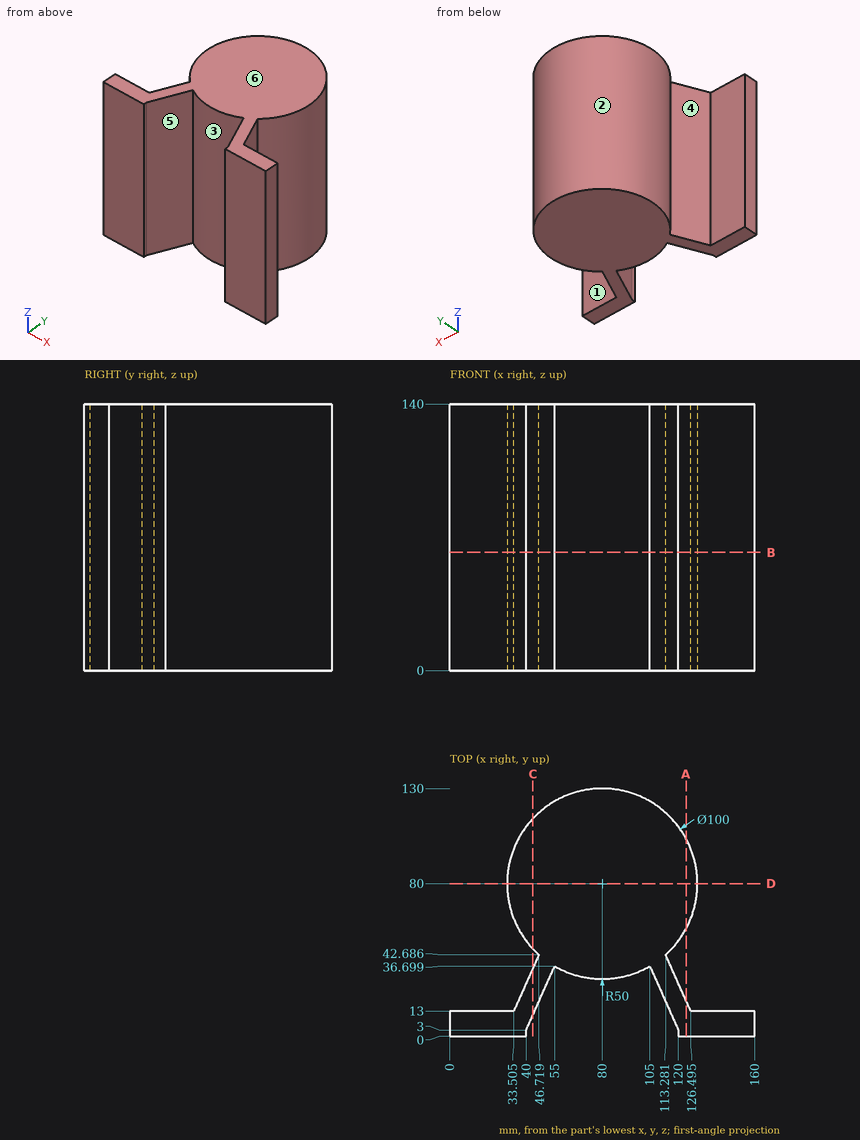
Geometry: see drawing. Coordinates: mm, zero at the bounding-box minimum. A direction names the side the tool comes from. Give positions to 0.01 mm unless a question says otherwise; leave off trailing zeros. Order: outer loops, then holes, each group sorted by start corner. A loop starts at its lowest first (then second) coordinate and runs counter-clockwise, first axis right, second up.
Q1. Set-up query: the marked faces 4, 5 and 6. Return all of +Z, -Z, +X, -X, +Y, -Y with unobstructed straight access to the full face (end or side cutting, diameter ignored); none if empty.
Checked values:
face 4: +Z, -Z, -X
face 5: +Z, -Z, -Y
face 6: +Z, +X, -X, +Y, -Y
Q2. Section C-C on x = 43.5. Output: boundary loops of the cut face in (y, z), and give its area (3 significant figures).
Checked values:
outline: (10.86, 0) - (35.45, 0) - (35.45, 140) - (10.86, 140) - close; (45.83, 0) - (114.17, 0) - (114.17, 140) - (45.83, 140) - close
area: 13,000 mm2
Q3. Ray query, probe 1 along X at (y, z) = (6, 12) (1 decimal); probe 2 along X at (y, z) = (23, 11) (1 decimal); probe 3 along X at (y, z) = (81, 45). Return the intervals inside material, ascending.
Checked values:
probe 1: x = 0 to 41.3, 118.7 to 160
probe 2: x = 38 to 48.9, 111.1 to 122
probe 3: x = 30.01 to 129.99
Q4. Section B-B on z = 62. Output: boundary loops of the cut face in (x, y) (1 decimal), and give its area (3 significant figures).
Checked values:
outline: (0, 0) - (40, 0) - (40, 3) - (55, 36.7) arc R50 ccw to (105, 36.7) - (120, 3) - (120, 0) - (160, 0) - (160, 13) - (126.5, 13) - (113.3, 42.7) arc R50 ccw (long way) to (46.7, 42.7) - (33.5, 13) - (0, 13) - close
area: 9,520 mm2
Q5. Section A-A on x = 124. Output: boundary loops of the cut face in (y, z) (1 decimal).
Checked values:
outline: (0, 0) - (18.6, 0) - (18.6, 140) - (0, 140) - close; (56.3, 0) - (103.7, 0) - (103.7, 140) - (56.3, 140) - close
Q6. Contact query for flat-ended pins moving along their axis: pin 1 Ø12 at (y, z) = (73.5, 112.5) entering from +X; pin 2 Ø5 at (x, z) = (113.5, 100) entering from +Y; pin 3 Ø1.5 at (y, z) = (115.5, 92.5) entering from +X. Output: stop coordinate, or through.
Checked values:
pin 1: stops at x = 130
pin 2: stops at y = 119.23
pin 3: stops at x = 115.95
Q7. Section D-D on y = 80. Output: boundary loops of the cut face in (x, z).
Checked values:
outline: (30, 0) - (130, 0) - (130, 140) - (30, 140) - close
Q8. Draft query along X for the marked faces 1, 2 and 3. Return one class per face: +X half, -X half, draft (parallel to the pull), parting line (faces both ways), or undercut.
Checked values:
face 1: draft
face 2: parting line
face 3: undercut
